from build123d import *

# Parameters (mm, degrees)
SKETCH1_R           = 3.3734375
BOSS_EXTRUDE1_DEPTH = 12.7


with BuildPart() as part:
    # Sketch1 → Boss-Extrude1 (new body)
    with BuildSketch(Plane(origin=(0, 0, 0), x_dir=(0, 0, -1), z_dir=(1, 0, 0))):
        with BuildLine():
            Line((0, -12.7), (0, -381))
            ThreePointArc((0, -381), (3.719743879, -389.980256121), (12.7, -393.7))
            Line((12.7, -393.7), (41.275, -393.7))
            ThreePointArc((41.275, -393.7), (50.255256121, -397.419743879), (53.975, -406.4))
            Line((53.975, -406.4), (53.975, -469.9))
            ThreePointArc((53.975, -469.9), (50.255256121, -478.880256121), (41.275, -482.6))
            Line((41.275, -482.6), (12.7, -482.6))
            ThreePointArc((12.7, -482.6), (3.719743879, -486.319743879), (0, -495.3))
            Line((0, -495.3), (0, -558.1424575))
            ThreePointArc((0, -558.1424575), (3.719743879, -567.122713621), (12.7, -570.8424575))
            Line((12.7, -570.8424575), (85.67674, -570.8424575))
            ThreePointArc((85.67674, -570.8424575), (88.621267556, -570.501864059), (91.410289955, -569.498071015))
            Line((91.410289955, -569.498071015), (167.095255646, -531.940375361))
            ThreePointArc((167.095255646, -531.940375361), (171.599093022, -529.093805409), (175.425396365, -525.386122262))
            Line((175.425396365, -525.386122262), (180.108605599, -519.804919463))
            Line((180.108605599, -519.804919463), (261.742877776, -422.517481393))
            Line((261.742877776, -422.517481393), (351.116781651, -316.006356758))
            ThreePointArc((351.116781651, -316.006356758), (359.938169615, -300.727331458), (363.001806424, -283.352647887))
            Line((363.001806424, -283.352647887), (363.001806424, -263.778902144))
            ThreePointArc((363.001806424, -263.778902144), (357.625647598, -241.034349984), (342.635087803, -223.103905101))
            Line((342.635087803, -223.103905101), (47.83309284, -2.531250739))
            ThreePointArc((47.83309284, -2.531250739), (44.233942259, -0.649416703), (40.224772495, 0))
            Line((40.224772495, 0), (12.7, 0))
            ThreePointArc((12.7, 0), (3.719743879, -3.719743879), (0, -12.7))
        make_face()
        with Locations((22.225, -22.225)):
            Circle(SKETCH1_R, mode=Mode.SUBTRACT)
        with Locations((22.225, -504.825)):
            Circle(SKETCH1_R, mode=Mode.SUBTRACT)
        with Locations((216.464615836, -288.472417571)):
            Circle(SKETCH1_R, mode=Mode.SUBTRACT)
        with Locations((134.830886903, -385.759530517)):
            Circle(SKETCH1_R, mode=Mode.SUBTRACT)
        with Locations((170.22785017, -511.513938695)):
            Circle(SKETCH1_R, mode=Mode.SUBTRACT)
        with Locations((251.862122347, -414.226500625)):
            Circle(SKETCH1_R, mode=Mode.SUBTRACT)
        with BuildLine():
            Line((81.631459634, -384.638877782), (87.754018145, -377.342309939))
            ThreePointArc((87.754018145, -377.342309939), (92.506625395, -376.926514968), (92.922420366, -381.679122218))
            Line((92.922420366, -381.679122218), (86.799861855, -388.975690061))
            ThreePointArc((86.799861855, -388.975690061), (82.047254605, -389.391485032), (81.631459634, -384.638877782))
        make_face(mode=Mode.SUBTRACT)
        with BuildLine():
            Line((211.291500366, -240.612602218), (205.168941855, -247.909170061))
            ThreePointArc((205.168941855, -247.909170061), (200.416334605, -248.324965032), (200.000539634, -243.572357782))
            Line((200.000539634, -243.572357782), (206.123098145, -236.275789939))
            ThreePointArc((206.123098145, -236.275789939), (210.875705395, -235.859994968), (211.291500366, -240.612602218))
        make_face(mode=Mode.SUBTRACT)
        with BuildLine():
            Line((288.55068278, -321.417631427), (282.428112367, -328.714189282))
            ThreePointArc((282.428112367, -328.714189282), (277.675504439, -329.129976501), (277.25971722, -324.377368573))
            Line((277.25971722, -324.377368573), (283.382287633, -317.080810718))
            ThreePointArc((283.382287633, -317.080810718), (288.134895561, -316.665023499), (288.55068278, -321.417631427))
        make_face(mode=Mode.SUBTRACT)
        with BuildLine():
            Line((80.03125722, -559.423888573), (86.153827633, -552.127330718))
            ThreePointArc((86.153827633, -552.127330718), (90.906435561, -551.711543499), (91.32222278, -556.464151427))
            Line((91.32222278, -556.464151427), (85.199652367, -563.760709282))
            ThreePointArc((85.199652367, -563.760709282), (80.447044439, -564.176496501), (80.03125722, -559.423888573))
        make_face(mode=Mode.SUBTRACT)
    extrude(amount=BOSS_EXTRUDE1_DEPTH)


solid = part.part
Can you work these out from the model? Positions are in its coordinate system, mm. A direction names the side the tool comes from. Coordinates: 2 decimals unless noted, no trailing zeros. Loops run counter-clockwise (first coordinate to the right, second up) from the corner with the lowest first, then second, coordinate; pieces in that order, holes last. Notation, with made-up numbers: (75.5, -28) - (120.5, -28) arc R28 cw to (120.5, -7) - close; hole circle Ø11 at (80, 24). An arc over 180 degrees is marked (long way). Put each result on its own line as item: value. Start each with the question number.
Item 1: Suppose I cut it at C-C (x = 2.75). State how many separate pieces and enclosed holes the cut face has, and give its area (3 significant figures).
Item 2: Suppose I cut it at A-A (z = -189.5). Please give me the cut outline in (x, y), and give its area (3 significant figures).
Item 3: Suppose I cut it at B-B (y = -199). Please give me the cut outline in (x, z).
Item 4: Which directions (+Z, -Z, +X, -X, +Y, -Y) give clear straight access to the entire face, cutting with the end or side of a thin tool? Please do faces 1 (the face through (6, -570.842, -49)), 2 (the face through (6.26, -389.88, -3.62)).
Item 5: If I drill on line 1 along Y through (x, z) = (6.75, -39.5); line 2 along Y through (x, z) = (2, -289); line 3 along Y through (x, z) = (11.5, -88.5), over which ranges is the centre line in solid material (lowest first)?
Item 6: If we mould it in two halves opening along Y, with no side actions, what happens to faces 3 (the face through (6.261, -114.362, -197.298)), 4 (the face through (6, -194, 0)), 5 (the face through (6.261, -397.322, -50.156))? For each: +Y half, -Y half, draft (parallel to the pull), parting line (faces both ways), or undercut.
Item 7: For pin 1 (5.5 mm diameter, centred on y = -288.47, z = -216.46, fed in from +X); pin 2 (1 mm diameter, centred on x = 10.5, z = -181.5, fed in from -Y); pin 3 (2 mm diameter, centred on x = 9.5, z = -247, fed in from -Y); pin 4 (6 mm diameter, centred on x = 3, z = -320.5, fed in from +Y), each with a flat end and sliding along its axis, tell me the tip position at first contact or that it passes through.
Here are the results:
1. separate pieces: 1
1. enclosed holes: 10
1. area: 132,000 mm²
2. outline: (0, -508.61) - (12.7, -508.61) - (12.7, -108.53) - (0, -108.53) - close
2. area: 5,080 mm²
3. outline: (0, -310.42) - (12.7, -310.42) - (12.7, 0) - (0, 0) - close
4. face 1: +Z, -Z, +X, -X, -Y
4. face 2: +Z, +X, -X
5. line 1: -570.84 to -482.6, -393.7 to 0
5. line 2: -390.03 to -320.72, -317.77 to -182.97
5. line 3: -570.53 to -559.83, -550.93 to -386.95, -376.68 to -32.96
6. face 3: +Y half
6. face 4: draft
6. face 5: undercut
7. pin 1: through
7. pin 2: y = -518.74
7. pin 3: y = -441.28
7. pin 4: y = -204.3
